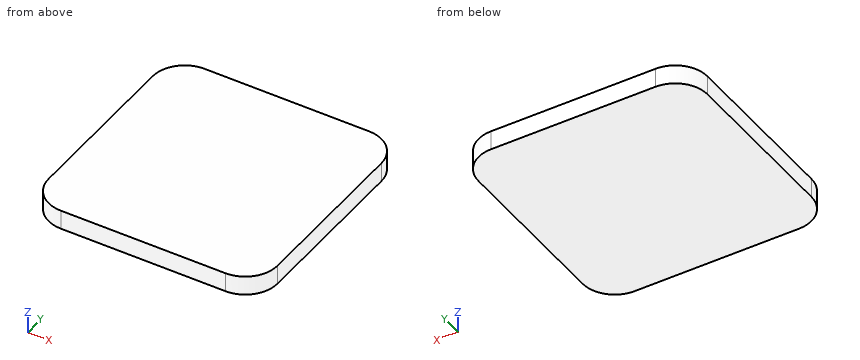
from build123d import *

# Parameters (mm, degrees)
BOSS_EXTRUDE1_DEPTH = 3


with BuildPart() as part:
    # Sketch2 → Boss-Extrude1 (new body)
    with BuildSketch(Plane.XY.offset(6)):
        with BuildLine():
            Line((-12.557097281, 18), (13, 18))
            ThreePointArc((13, 18), (16.535533906, 16.535533906), (18, 13))
            Line((18, 13), (18, -13))
            ThreePointArc((18, -13), (16.535533906, -16.535533906), (13, -18))
            Line((13, -18), (-12.557097281, -18))
            ThreePointArc((-12.557097281, -18), (-16.092631187, -16.535533906), (-17.557097281, -13))
            Line((-17.557097281, -13), (-17.557097281, 13))
            ThreePointArc((-17.557097281, 13), (-16.092631187, 16.535533906), (-12.557097281, 18))
        make_face()
    extrude(amount=BOSS_EXTRUDE1_DEPTH)


solid = part.part
The model under review builds one solid part; all positions refer to its coordinate system, in mm. Coordinates: 2 decimals unless noted, no trailing zeros. Write each loop counter-clockwise with the first axis right and the second up, starting at its lowest first coordinate (ties: lowest second). Pieces come first, ordered by that corner, then holes. Notation, with made-up numbers: M 49,20.25 L 89,20.25 A19 ccw 89,52.25 Z; hole C -39.75,33 d8. An arc over 180 degrees is marked long. Put each result on its own line as item: value.
1) Add section B-B on y = -15. Give the boundary of the cut face in (x, z).
Computed:
outline: M -17.14,6 L 17.58,6 L 17.58,9 L -17.14,9 Z
2) Wall thickness on probe 1 along Y at (x, z) = (-14.5, 6.45); probe 2 along X at (y, z) = (-15.5, 7.7); probe 3 along X at (y, z) = (15, 8.3): over which ranges is each line inside the solid? List them lowest first. Write a range as [from, to].
Computed:
probe 1: y = [-17.61, 17.61]
probe 2: x = [-16.89, 17.33]
probe 3: x = [-17.14, 17.58]
3) Add section A-A on z = 7.8. Give the boundary of the cut face in (x, y).
Computed:
outline: M -17.56,-13 A5 ccw -12.56,-18 L 13,-18 A5 ccw 18,-13 L 18,13 A5 ccw 13,18 L -12.56,18 A5 ccw -17.56,13 Z
